Print and shaded views of the part. All mm, measured from the part's lowest x, y and z. A direction names the side the tool comes from. Give positions to 0.01 mm unless a question says otherwise; leave off trailing zeros. Loops run counter-clockwise (first coordinate to the right, second up) from the corner with the lowest first, then second, coordinate; pieces in that order, holes last. Notation, with made-up numbers: M 69,47 L 126,47 A17 ccw 126,65 Z; hole C 3,12.25 d2. An arc over 180 degrees is marked long. Answer in a Markdown table with one row per item.
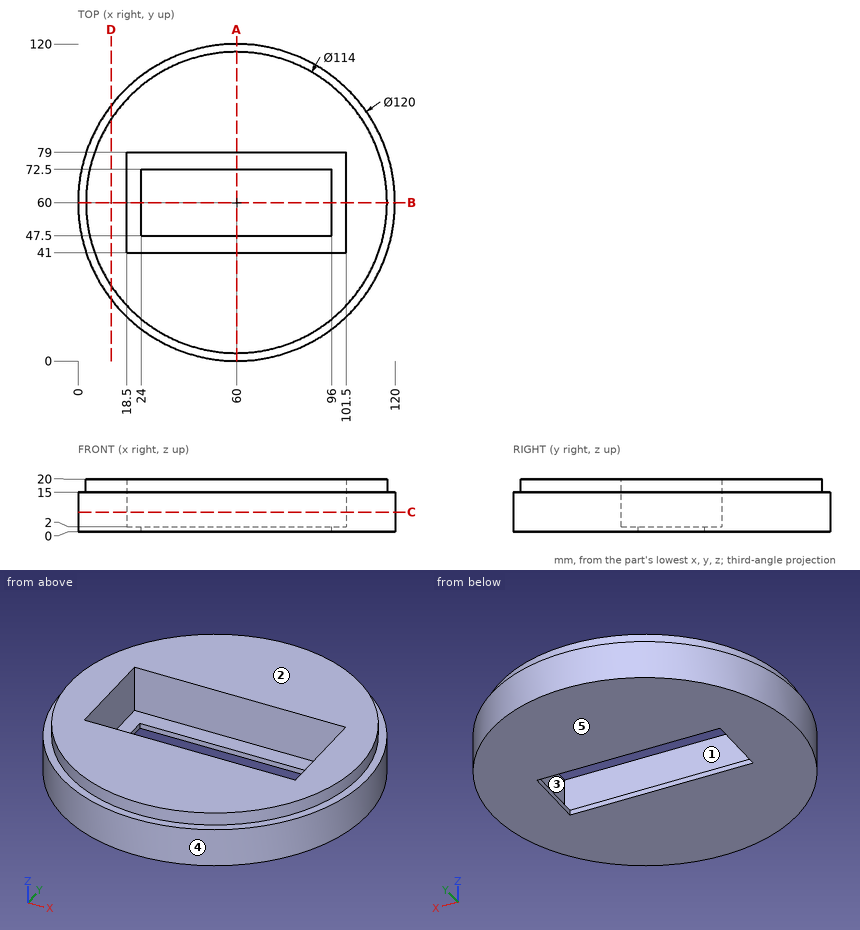
(1) Saw through at B-B, the plane y = 60. Give the cut face in (x, z), and give its area (3 significant figures).
Established:
| item | result |
|---|---|
| outline | M 0,0 L 24,0 L 24,2 L 18.5,2 L 18.5,20 L 3,20 L 3,15 L 0,15 Z; M 96,0 L 120,0 L 120,15 L 117,15 L 117,20 L 101.5,20 L 101.5,2 L 96,2 Z |
| area | 732 mm2 |
(2) Mould opens along Y. For the marked faces 3, 4 and 5 say: pulls with the +Y half, pulls with the -Y half, needs draft (parallel to the pull), parting line crosses it, or undercut.
Established:
| item | result |
|---|---|
| face 3 | undercut |
| face 4 | parting line crosses it |
| face 5 | needs draft |
(3) Wall check: L1, parallel to Y at x = 68, z = 13.75; L2, parallel to Y at x = 24, z = 7.5; L3, parallel to X at y = 66, z = 12.25. Give the ranges that are in metal, low to high.
Established:
| item | result |
|---|---|
| L1 | y = 0.54 to 41, 79 to 119.46 |
| L2 | y = 12 to 41, 79 to 108 |
| L3 | x = 0.3 to 18.5, 101.5 to 119.7 |
(4) Saw through at A-A, the plane x = 60. Give the cut face in (y, z).
Established:
| item | result |
|---|---|
| outline | M 0,0 L 47.5,0 L 47.5,2 L 41,2 L 41,20 L 3,20 L 3,15 L 0,15 Z; M 72.5,0 L 120,0 L 120,15 L 117,15 L 117,20 L 79,20 L 79,2 L 72.5,2 Z |
(5) Flat gauge pins, fed straight in: P1, Ø1.5, axis at x = 72, z = 6, coming from the +Y side; P2, Ø9, axis at y = 65.5, z = 9.5, coming from the +X side; P3, Ø1, axis at x = 54.5, z = 2.5, coming from the +Y side; P4, Ø10, axis at x = 32.5, y = 63.5, coming from the -Z side. Where does each tip first touch, or does it go through?
Established:
| item | result |
|---|---|
| P1 | stops at y = 118.94 |
| P2 | stops at x = 119.99 |
| P3 | stops at y = 119.79 |
| P4 | passes through |
(6) Which spindle directions (+Z, -Z, +X, -X, +Y, -Y) get a long thin tool onto all of the face, cutting with end or side? Do the marked faces 1 and 2. Say none if no direction does.
Established:
| item | result |
|---|---|
| face 1 | +Z |
| face 2 | +Z, +X, -X, +Y, -Y |
(7) Saw through at C-C, the plane z = 7.5. Give the cut face in (x, y).
Established:
| item | result |
|---|---|
| outline | C 60,60 d120; hole M 18.5,41 L 101.5,41 L 101.5,79 L 18.5,79 Z |
(8) Saw through at D-D, the plane x = 12.5. Give the cut face in (y, z), and give its area (3 significant figures).
Established:
| item | result |
|---|---|
| outline | M 23.34,0 L 96.66,0 L 96.66,15 L 91.51,15 L 91.51,20 L 28.49,20 L 28.49,15 L 23.34,15 Z |
| area | 1,410 mm2 |
